Geometry: see drawing. Coordinates: mm, zero at the bounding-box minimum. A direction names the side the tool comes from. Round coordinates to 2 decimals unless told otherwise and drop trailing zeros. Order: outer loops, then holes, each group sorted by start corner. A loop starts at its lowest first (then second) coordinate and runs counter-clockwise, first axis right, second up. Notation, with made-up numbers: (-25, 73) -> (13, 73) arc R21 cw to (13, 110) -> close; hole circle Ø6 at (59.25, 1). An arc over 180 degrees is marked (long way). Write item = value, one per line. Start each with the question number.
(1) Ray query, line 1 (Y direction, x = 13, z = 80.5); line 2 (Y direction, x = 4, z = 15); line 3 (X direction, y = 5, z = 16.5). Return the intervals inside material, ascending.
(2) Cut plane A-A on x = 2.5. Return the cut outline in (y, z) (1 decimal), then the cut area to 3 significant figures.
(3) Contact query for flat-ended pins moving along their axis: pin 1 Ø5 at (x, z) = (13, 59.5) entering from +Y; pin 2 Ø6 at (y, z) = (12, 11.5) entering from +X; pin 3 Ø1.5 at (y, z) = (18, 49) entering from -X. Output: stop coordinate, or through.
(4) Draft query along Y for the marked faces 1, 2, 3 and 4. Return one class per face: released by +Y, released by -Y, zero draft, split by the parting line, or undercut.
(5) Reachability of the marked faces 5 and 6 from +Z, -Z, +X, -X, +Y, -Y: full face, straight path, thin tool, end or side. Return the list, or none.
(6) Cut plane D-D on x = 8. Return the cut outline in (y, z) (1 decimal).
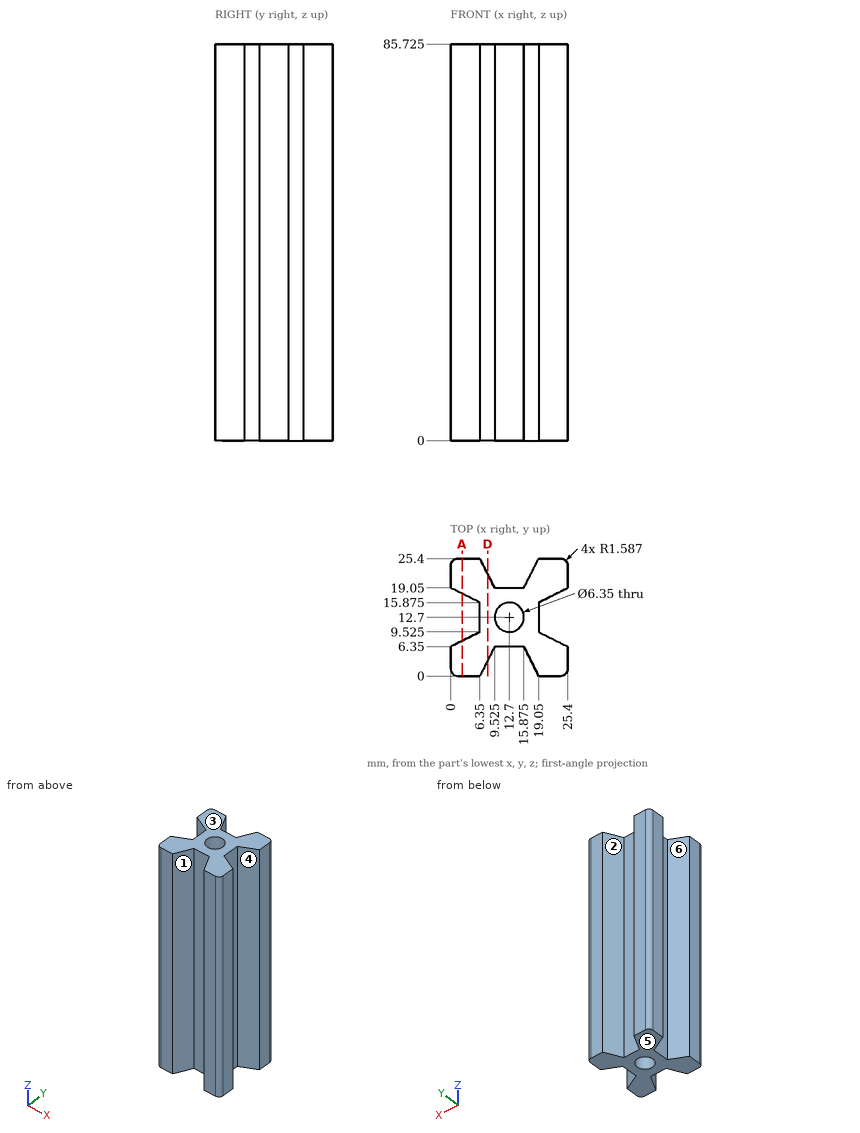
Evaluation:
q1.line_1 = 6.35 to 9.54, 15.86 to 19.05
q1.line_2 = 0 to 8.35, 17.05 to 25.4
q1.line_3 = 0 to 8.85, 16.55 to 25.4
q2.outline = (0, 0) -> (7.6, 0) -> (7.6, 85.7) -> (0, 85.7) -> close; (17.8, 0) -> (25.4, 0) -> (25.4, 85.7) -> (17.8, 85.7) -> close
q2.area = 1,300 mm^2
q3.pin_1 = 19.05
q3.pin_2 = 20.1
q3.pin_3 = 0.6
q4.face_1 = released by -Y
q4.face_2 = released by +Y
q4.face_3 = zero draft
q4.face_4 = undercut
q5.face_5 = -Z, +X, -X, +Y, -Y
q5.face_6 = +Z, -Z, -X
q6.outline = (3.3, 0) -> (22.1, 0) -> (22.1, 85.7) -> (3.3, 85.7) -> close
